from build123d import *

# Parameters (mm, degrees)
SKETCH_1_R      = 1.75
EXTRUDE_1_DEPTH = 1.2


with BuildPart() as part:
    # 草图1 → 凸台-拉伸1 (new body)
    with BuildSketch(Plane.XZ):
        with BuildLine():
            Line((6.5, -20.5), (6.5, 20.5))
            ThreePointArc((6.5, 20.5), (0, 27), (-6.5, 20.5))
            Line((-6.5, 20.5), (-6.5, -20.5))
            ThreePointArc((-6.5, -20.5), (0, -27), (6.5, -20.5))
        make_face()
        with Locations(Location((0, 19.85, 0), (0, 0, 90))):
            Circle(SKETCH_1_R, mode=Mode.SUBTRACT)
        with Locations(Location((0, -19.85, 0), (0, 0, 90))):
            Circle(SKETCH_1_R, mode=Mode.SUBTRACT)
    extrude(amount=-EXTRUDE_1_DEPTH)


solid = part.part
Work out the finished part from the listing and answer in its coordinate system (mm). Give positions to 0.01 mm unless a question says otherwise; leave off trailing zeros. Write each loop counter-clockwise with the first axis right and the second up, starting at its lowest first coordinate (ties: lowest second). Pieces come first, ordered by that corner, then holes. Notation, with made-up numbers: M 66.25,16.5 L 94.25,16.5 A9 cw 94.25,23.5 Z; hole C -17,48 d3. An arc over 180 degrees is marked long. Answer as CSV lines item,"result".
Q1. A cutting plane is placed at C-C on y = 0.8. Write down the section's boundary in (x, z), plus the area to 3 significant figures.
A:
outline,"M -6.5,-20.5 A6.5 ccw 6.5,-20.5 L 6.5,20.5 A6.5 ccw -6.5,20.5 Z; hole C 0,-19.85 d3.5; hole C 0,19.85 d3.5"
area,"646 mm²"
Q2. A cutting plane is placed at A-A on x = 0. Write down the section's boundary in (y, z), plus the area to 3 significant figures.
A:
outline,"M 0,-27 L 1.2,-27 L 1.2,-21.6 L 0,-21.6 Z; M 0,-18.1 L 1.2,-18.1 L 1.2,18.1 L 0,18.1 Z; M 0,21.6 L 1.2,21.6 L 1.2,27 L 0,27 Z"
area,"56.4 mm²"
Q3. A cutting plane is placed at B-B on z = 19.85. Write down the section's boundary in (x, y).
A:
outline,"M -6.5,0 L -1.75,0 L -1.75,1.2 L -6.5,1.2 Z; M 1.75,0 L 6.5,0 L 6.5,1.2 L 1.75,1.2 Z"
Q4. Find the intervals of material crossed by probe 1 along X at (y, z) = (0.8, 19.85); probe 2 along Z at (x, y) = (0.5, 0.85); probe 3 along Z at (x, y) = (-1, 0.35), in increasing order. Write a range as [from, to].
A:
probe 1,"x = [-6.5, -1.75], [1.75, 6.5]"
probe 2,"z = [-26.98, -21.53], [-18.17, 18.17], [21.53, 26.98]"
probe 3,"z = [-26.92, -21.29], [-18.41, 18.41], [21.29, 26.92]"
Q5. A cutting plane is placed at D-D on z = -22.5. Write down the section's boundary in (x, y).
A:
outline,"M -6.18,0 L 6.18,0 L 6.18,1.2 L -6.18,1.2 Z"
Q6. Given P1, Ø6, axis at x = -2.5, z = 4, coming from the -Y side; P2, Ø3, axis at x = 0, z = 19.85, coming from the +Y side, each flat-ended and moving along its own axis, determine where each tip first touches the part or whether it passes through.
A:
P1,"stops at y = 0"
P2,"passes through"
Q7. The mould has two halves that part along X. Classify faces 1 (the flat face through (-6.5, 1, 0)), 2 (the cylindrical face through (0, 1, 27)), 3 (the cylindrical face through (-0.08, 0.59, -21.6)): +X half, -X half, draft (parallel to the pull), parting line (faces both ways), or undercut.
A:
face 1,"-X half"
face 2,"parting line"
face 3,"undercut"
